Verification items for the finished model (mm, model axes). A direction names the side the tool comes from. Give positions to 0.01 mm unless a question says otherwise; leave off trailing zeros. Order: outer loops, then holes, each group sorted by start corner. A loop starts at its lowest first (then second) coordinate and runs counter-clockwise, first axis right, second up. Notation, with made-up numbers: (60, 75.25) -> (72, 75.25) arc R21 ccw to (72, 105.25) -> close; hole circle Ø9 at (29, 22). An arc over 180 degrees is marked (long way). Return JSON: item names as keys, results as strings. Group by question number.
(1) Cross-section at B-B on x = -10.25. Enter the section's corners in (y, z), then the cut area to 3 significant figures.
(2) Release check for a two-part mould opening along Y. For faces 1 (the face through (-10, 2.54, -4)), 2 (the face through (0, 1, -4)), 3 (the face through (-6, 0.71, -3)) record: pulls with the +Y half, pulls with the -Y half, needs draft (parallel to the pull), parting line crosses it, or undercut.
(3) Depth check by flat-ended pin: pin 1 Ø1 at (x, z) = (-10, -3.5) entering from -Y. Enter the tip coordinate at first touch or a pass-through.
(4) Cross-section at C-C on y = 1.35. State how many separate pieces and enclosed holes the cut face has, then the cut area to 3 significant figures.
(5) Tool access check on faces 4 (the face through (-11.93, 0.9, -2.6)), 5 (the face through (-15.8, 1.11, -5.4)), 6 (the face through (-10, 1, -7.5)). Record the directions out of +Z, -Z, +X, -X, +Y, -Y that give a thin tool (end or side, any length) a straight path to the whole face; none if there is none.
(6) Thickness scan on line 1 along Y through (x, z) = (-3.25, -6.75); line 2 along Y through (x, z) = (-6.5, -1.75); line 3 along Z through (x, y) = (-11, 0.9). Record the ranges inside material, lowest first.
(7) Cross-section at A-A on z = -7.75. Enter the section's corners in (x, y), then the cut area to 3 significant figures.
from build123d import *

# Parameters (mm, degrees)
BOSS_EXTRUDE1_DEPTH = 20.32
SKETCH2_W           = 2
SKETCH2_H           = 0.6
CUT_EXTRUDE1_DEPTH  = 5.5
SKETCH3_W           = 1
SKETCH3_H           = 1
CUT_EXTRUDE2_DEPTH  = 6
SKETCH4_W           = 2
SKETCH4_H           = 2
CUT_EXTRUDE3_DEPTH  = 0.5
CUT_EXTRUDE3_TAPER  = 45
LPATTERN1_COUNT     = 8
LPATTERN1_PITCH     = 2.54


with BuildPart() as part:
    # Sketch1 → Boss-Extrude1 (new body)
    with BuildSketch(Plane(origin=(0, 0, 0), x_dir=(0, 0, -1), z_dir=(1, 0, 0))):
        Polygon((8.5, 2.54), (0, 2.54), (0, 0), (8.5, 0), (8.5, 0.75), (7.5, 0.75), (7.5, 1.709993), (8.5, 1.709993), align=None)
    extrude(amount=-BOSS_EXTRUDE1_DEPTH)

    # Sketch2 → Cut-Extrude1 (cut)
    with BuildSketch(Plane(origin=(0, 0, -7.5), x_dir=(-1, 0, 0), z_dir=(0, 0, -1))):
        with Locations((1.27, 1.409993)):
            Rectangle(SKETCH2_W, SKETCH2_H)
    cut_extrude1 = extrude(amount=-CUT_EXTRUDE1_DEPTH, mode=Mode.SUBTRACT)

    # Sketch3 → Cut-Extrude2 (cut)
    with BuildSketch(Plane(origin=(0, 0, 0), x_dir=(-1, 0, 0), z_dir=(0, 0, -1))):
        with Locations((1.27, 1.209993)):
            Rectangle(SKETCH3_W, SKETCH3_H)
    cut_extrude2 = extrude(amount=CUT_EXTRUDE2_DEPTH, mode=Mode.SUBTRACT)

    # Sketch4 → Cut-Extrude3 (cut)
    with BuildSketch(Plane.XY):
        with Locations((-1.27, 1.209993)):
            Rectangle(SKETCH4_W, SKETCH4_H)
    cut_extrude3 = extrude(amount=-CUT_EXTRUDE3_DEPTH, taper=CUT_EXTRUDE3_TAPER, mode=Mode.SUBTRACT)

    # LPattern1: Cut-Extrude1, Cut-Extrude2, Cut-Extrude3 ×8
    with Locations(*[(-i * LPATTERN1_PITCH, 0, 0) for i in range(1, LPATTERN1_COUNT)]):
        add(cut_extrude1, mode=Mode.SUBTRACT)
        add(cut_extrude2, mode=Mode.SUBTRACT)
        add(cut_extrude3, mode=Mode.SUBTRACT)


solid = part.part
Verdict:
{
 "1": {"outline": "(0, -8.5) -> (0.75, -8.5) -> (0.75, -7.5) -> (1.71, -7.5) -> (1.71, -8.5) -> (2.54, -8.5) -> (2.54, 0) -> (0, 0) -> close", "area": "20.6 mm²"},
 "2": {"face 1": "pulls with the +Y half", "face 2": "needs draft", "face 3": "undercut"},
 "3": {"pin 1": "y = 0"},
 "4": {"separate pieces": "9", "enclosed holes": "0", "area": "46.4 mm²"},
 "5": {"face 4": "+Z", "face 5": "-Z", "face 6": "-Z, +X, -X"},
 "6": {"line 1": "0 to 1.11, 1.71 to 2.54", "line 2": "0 to 0.71, 1.71 to 2.54", "line 3": "-7.5 to -6"},
 "7": {"outline": "(-20.32, 0) -> (0, 0) -> (0, 0.75) -> (-20.32, 0.75) -> close; (-20.32, 1.71) -> (0, 1.71) -> (0, 2.54) -> (-20.32, 2.54) -> close", "area": "32.1 mm²"}
}
